The listing builds one solid part. Answer for the finished solid, in the listing's coordinates (mm). A direction names the side the tool comes from. Give positions to 0.01 mm unless a question says otherwise; leave off trailing zeros. Order: outer loops, then holes, each group sorted by start corner. A loop starts at its lowest first (then second) coordinate and runs counter-clockwise, first axis right, second up. Notation, with made-up numbers: (-38, 54) -> (-18, 54) arc R35 ccw to (-18, 88) -> close; hole circle Ø4 at (38, -30.75). An arc over 180 degrees is marked (long way). One line per question, with ' | ' between items. Start each with the question number.
```python
from build123d import *

# Parameters (mm, degrees)
F1_DEPTH = 1104.9


with BuildPart() as f1:
    # F0 (on Right) → F1 (new body)
    with BuildSketch(Plane.YZ):
        with BuildLine():
            Line((76.2, 0), (-76.2, 0))
            Line((-76.2, 0), (-76.2, -63.4238))
            ThreePointArc((-76.2, -63.4238), (-72.574321, -62.102069), (-70.649887, -58.757061))
            Line((-70.649887, -58.757061), (-63.124886, -15.566335))
            ThreePointArc((-63.124886, -15.566335), (-59.952782, -10.052651), (-53.976459, -7.874))
            Line((-53.976459, -7.874), (53.976459, -7.874))
            ThreePointArc((53.976459, -7.874), (59.952782, -10.052651), (63.124886, -15.566335))
            Line((63.124886, -15.566335), (70.649887, -58.757061))
            ThreePointArc((70.649887, -58.757061), (72.574321, -62.102069), (76.2, -63.4238))
            Line((76.2, -63.4238), (76.2, 0))
        make_face()
    extrude(amount=F1_DEPTH)


solid = f1.part
```
(1) For faces 4 (the face through (544.716, 66.835, -36.859)), 5 (the face through (545, 1, 0)), determine the directions among +Z, -Z, +X, -X, +Y, -Y from which every point of the face is accessible in a straight line to the end or side of a thin tool.
(2) Consider line 1 (Y direction, x = 697, z = -12); line 2 (Y direction, x = 777.5, z = -61); line 3 (Z direction, x = 549.5, y = 29). Determine where each line is inside the solid, lowest interval first.
(3) The part is cut by section C-C on y = 0.5. Determine the outline of the cut face in (x, z), plus the area to 3 significant figures.
(4) The part is cut by section B-B on x = 427. Determine the outline of the cut face in (y, z), plus the area to 3 significant figures.
(5) Determine the mould class of faces 1 (the face through (1104.9, 0, -6)), 2 (the face through (545, -76.2, -31)), 3 (the face through (544.72, -66.94, -37.46)) for opening direction Y: pulls with the +Y half, pulls with the -Y half, needs draft (parallel to the pull), parting line crosses it, or undercut.
(6) The part is cut by section A-A on z = -37. Determine the outline of the cut face in (x, y).
(7) Given P1, Ø1, axis at x = 555.5, y = 5.5, coming from the -Z side, flat-ended and moving along its own axis, determine where the tip first touches the part or whether it passes through.
Result sheet:
1) face 4: -Z, +X, -X | face 5: +Z, +X, -X, +Y, -Y
2) line 1: y = -76.2 to -61.7, 61.7 to 76.2 | line 2: y = -76.2 to -71.57, 71.57 to 76.2 | line 3: z = -7.87 to 0
3) outline: (0, -7.87) -> (1104.9, -7.87) -> (1104.9, 0) -> (0, 0) -> close | area: 8,700 mm^2
4) outline: (-76.2, -63.42) arc R5.63 ccw to (-70.65, -58.76) -> (-63.12, -15.57) arc R9.29 cw to (-53.98, -7.87) -> (53.98, -7.87) arc R9.29 cw to (63.12, -15.57) -> (70.65, -58.76) arc R5.63 ccw to (76.2, -63.42) -> (76.2, 0) -> (-76.2, 0) -> close | area: 2,280 mm^2
5) face 1: needs draft | face 2: pulls with the -Y half | face 3: undercut
6) outline: (0, -76.2) -> (1104.9, -76.2) -> (1104.9, -66.86) -> (0, -66.86) -> close; (0, 66.86) -> (1104.9, 66.86) -> (1104.9, 76.2) -> (0, 76.2) -> close
7) P1: stops at z = -7.87
